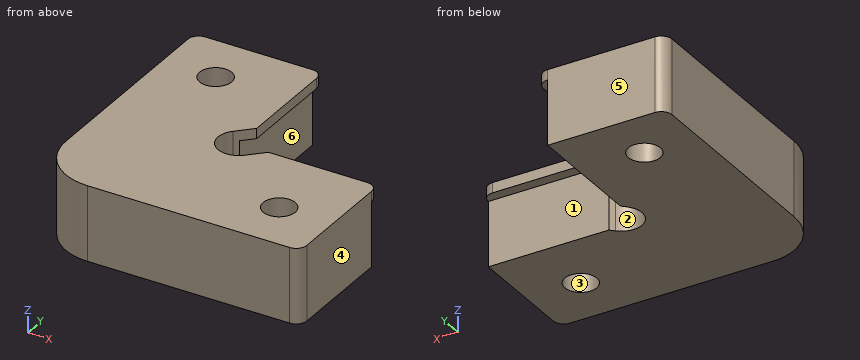
```python
from build123d import *

# Parameters (mm, degrees)
SKETCH1_R           = 1.5
BOSS_EXTRUDE1_DEPTH = 7
BOSS_EXTRUDE2_DEPTH = 0.95


with BuildPart() as part:
    # Sketch1 → Boss-Extrude1 (new body)
    with BuildSketch(Plane.XY):
        with BuildLine():
            Line((-11, 13.003727625), (-11, -5.867758287))
            ThreePointArc((-11, -5.867758287), (-9.496801205, -9.496801205), (-5.867758287, -11))
            Line((-5.867758287, -11), (13.003727625, -11))
            ThreePointArc((13.003727625, -11), (13.708198577, -10.708198577), (14, -10.003727625))
            Line((14, -10.003727625), (14, 0))
            Line((14, 0), (2.757716447, 0))
            Line((2.757716447, 0), (2.382592719, -0.375123728))
            ThreePointArc((2.382592719, -0.375123728), (-0.375123728, -0.375123728), (-0.375123728, 2.382592719))
            Line((-0.375123728, 2.382592719), (0, 2.757716447))
            Line((0, 2.757716447), (0, 14))
            Line((0, 14), (-10.003727625, 14))
            ThreePointArc((-10.003727625, 14), (-10.708198577, 13.708198577), (-11, 13.003727625))
        make_face()
        with Locations((9, -6)):
            Circle(SKETCH1_R, mode=Mode.SUBTRACT)
        with Locations((-6, 9)):
            Circle(SKETCH1_R, mode=Mode.SUBTRACT)
    extrude(amount=BOSS_EXTRUDE1_DEPTH)

    # Sketch2 → Boss-Extrude2 (add)
    with BuildSketch(Plane.XY.offset(7)):
        with BuildLine():
            Line((2.757716447, 0), (3.757716447, 1))
            Line((3.757716447, 1), (13, 1))
            ThreePointArc((13, 1), (13.707106781, 0.707106781), (14, 0))
            Line((14, 0), (2.757716447, 0))
        make_face()
        with BuildLine():
            Line((0, 2.757716447), (1, 3.757716447))
            Line((1, 3.757716447), (1, 13))
            ThreePointArc((1, 13), (0.707106781, 13.707106781), (0, 14))
            Line((0, 14), (0, 2.757716447))
        make_face()
    extrude(amount=-BOSS_EXTRUDE2_DEPTH)


solid = part.part
```
For this review, take the finished solid that the model builds, in its own axes (mm). Face numbers are marked on the shaded views. A direction names the side the tool comes from. Round coordinates to 2 decimals unless told otherwise and drop trailing zeros. Write each loop counter-clockwise with the first axis right and the second up, starting at its lowest first coordinate (ties: lowest second). Pieces come first, ordered by that corner, then holes. Notation, with made-up numbers: (33, 47.25) - (57, 47.25) arc R23 ccw to (57, 61.25) - close; hole circle Ø10 at (64.25, 19.5). An arc over 180 degrees is marked (long way). Use CSV: the item, a comma, the result in double quotes.
1) Add section C-C on y = 6.75. Write out the cut boundary in (x, z).
Conclusion:
outline,"(-11, 0) - (0, 0) - (0, 6.05) - (1, 6.05) - (1, 7) - (-11, 7) - close"
2) The part is to be moulded in two halves that separate along Y. For the marked faces 1, 2, 3 and 4, say which applies: pulls with the +Y half, pulls with the -Y half, needs draft (parallel to the pull), parting line crosses it, or undercut.
Conclusion:
face 1,"pulls with the +Y half"
face 2,"undercut"
face 3,"undercut"
face 4,"needs draft"
3) Wall thickness on line 1 along Y through (x, z) = (-6, 5.25); line 2 along Y through (x, z) = (9, 1.5); line 3 along X through (y, z) = (12, 4.5): over which ranges is each line inside the solid? List them lowest first. Write a range as from..to.
Conclusion:
line 1,"y = -11..7.5, 10.5..14"
line 2,"y = -11..-7.5, -4.5..0"
line 3,"x = -11..0"
4) Clearance check with flat-ended pins moving along their axes: pin 1 Ø1.8 at (x, z) = (10.5, 3.5) entering from +Y; pin 2 Ø0.8 at (x, z) = (9, 7) entering from +Y; pin 3 Ø1 at (x, y) = (3.5, 1.5) entering from -Z; pin 4 Ø0.5 at (x, y) = (7, 0.5) entering from -Z. State where each tip first meets the part, or that it passes through.
Conclusion:
pin 1,"stops at y = 0"
pin 2,"stops at y = 1"
pin 3,"passes through"
pin 4,"stops at z = 6.05"
5) Add section A-A on x = 9. Write out the cut boundary in (y, z), and give its area (4 significant figures).
Conclusion:
outline,"(-11, 0) - (-7.5, 0) - (-7.5, 7) - (-11, 7) - close; (-4.5, 0) - (0, 0) - (0, 6.05) - (1, 6.05) - (1, 7) - (-4.5, 7) - close"
area,"56.95 mm^2"
6) Add section B-B on z = 1.25. Write out the cut boundary in (x, y), and give its area (3 significant figures).
Conclusion:
outline,"(-11, -5.87) arc R5.13 ccw to (-5.87, -11) - (13, -11) arc R1 ccw to (14, -10) - (14, 0) - (2.76, 0) - (2.38, -0.38) arc R1.95 cw to (-0.38, 2.38) - (0, 2.76) - (0, 14) - (-10, 14) arc R1 ccw to (-11, 13) - close; hole circle Ø3 at (-6, 9); hole circle Ø3 at (9, -6)"
area,"405 mm^2"
7) For the marked faces 5 and 6, list the 3-axis set-ups (+Z, -Z, +X, -X, +Y, -Y) from which the entire face can be reached by the end or side of a thin tool; tool diameter is ignored.
Conclusion:
face 5,"+Z, -Z, +X, -X, +Y"
face 6,"-Z, +X, +Y"
8) Add section D-D on y = 10. Write out the cut boundary in (x, z), and give its area (3 significant figures).
Conclusion:
outline,"(-11, 0) - (-7.12, 0) - (-7.12, 7) - (-11, 7) - close; (-4.88, 0) - (0, 0) - (0, 6.05) - (1, 6.05) - (1, 7) - (-4.88, 7) - close"
area,"62.3 mm^2"
